CAD build for the part. Positions are in the model's coordinates, mm. Face numbers are marked on the shaded views. A direction names the side the tool comes from. Give positions to 0.01 mm unless a question says otherwise; leave off trailing zeros. Write each loop counter-clockwise with the first axis right and the second up, starting at its lowest first coordinate (ties: lowest second). Pieces come first, ordered by that corner, then holes. Notation, with made-up numbers: (8, 84) -> (43, 84) arc R23 cw to (43, 108) -> close; hole circle Ø11 at (-10.5, 48.5). An arc over 180 degrees is marked (long way). Answer as a JSON object with one key per item and string values.
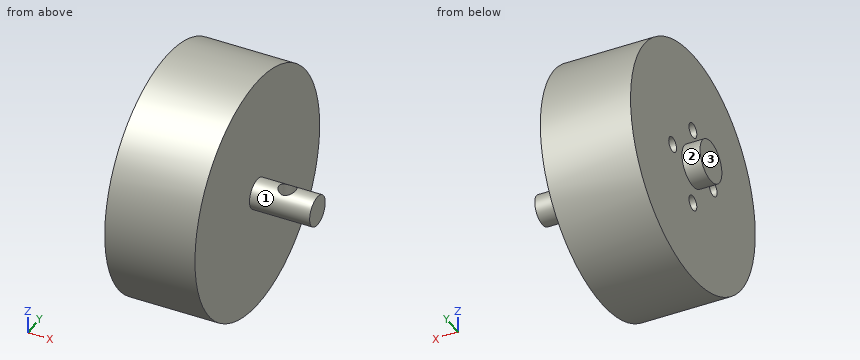
```python
from build123d import *

# Parameters (mm, degrees)
SKETCH_1_R               = 3.5
EXTRUDE_1_DEPTH          = 3
SKETCH_2_R               = 20
EXTRUDE_2_DEPTH          = 15
SKETCH_3_R               = 2.5
EXTRUDE_3_DEPTH          = 10
CUT_EXTRUDE_1_DEPTH      = 10
CUT_EXTRUDE_1_DEPTH_BACK = 10
SKETCH_4_R               = 1.4
HOLE_WIZARD_M3_1_D       = 2.5
HOLE_WIZARD_M3_1_DEPTH   = 6.748924226
HOLE_WIZARD_M3_1_TIP     = 0.751075774


with BuildPart() as part:
    # 草图1 → 凸台-拉伸1 (new body)
    with BuildSketch(Plane(origin=(0, 0, 0), x_dir=(0, 0, -1), z_dir=(1, 0, 0))):
        Circle(SKETCH_1_R)
    extrude(amount=EXTRUDE_1_DEPTH)

    # 草图2 → 凸台-拉伸2 (add)
    with BuildSketch(Plane(origin=(3, 0, 0), x_dir=(0, 0, -1), z_dir=(1, 0, 0))):
        Circle(SKETCH_2_R)
    extrude(amount=EXTRUDE_2_DEPTH)

    # 草图3 → 凸台-拉伸3 (add)
    with BuildSketch(Plane(origin=(18, 0, 0), x_dir=(0, 0, -1), z_dir=(1, 0, 0))):
        Circle(SKETCH_3_R)
    extrude(amount=EXTRUDE_3_DEPTH)

    # 草图4 → 切除-拉伸1 (cut, two sides: drawn at the far end of the back side and taken through both)
    with BuildSketch(Plane.XY.offset(-CUT_EXTRUDE_1_DEPTH_BACK)):
        with Locations((23, 0)):
            Circle(SKETCH_4_R)
    extrude(amount=CUT_EXTRUDE_1_DEPTH + CUT_EXTRUDE_1_DEPTH_BACK, mode=Mode.SUBTRACT)

    # M3 螺纹孔1
    with Locations(Plane(origin=(3, 0, 6.5), x_dir=(0, 0, -1), z_dir=(-1, 0, 0))):
        with Locations((0, 0), (6.5, 6.5), (13, 0), (6.5, -6.5)):
            Hole(HOLE_WIZARD_M3_1_D / 2, depth=HOLE_WIZARD_M3_1_DEPTH)
            with Locations((0, 0, -(HOLE_WIZARD_M3_1_DEPTH + HOLE_WIZARD_M3_1_TIP / 2))):  # 118° drill point
                Cone(0, HOLE_WIZARD_M3_1_D / 2, HOLE_WIZARD_M3_1_TIP, mode=Mode.SUBTRACT)


solid = part.part
```
1) Wall check: probe 1 along Y at (x, z) = (4.75, 0); probe 2 along Y at (x, z) = (8.75, 1); probe 3 along X at (y, z) = (6.5, 12.5). Give the ranges that are in metal, low to high.
Model answer:
{"probe 1": "y = -20 to -7.75, -5.25 to 5.25, 7.75 to 20", "probe 2": "y = -19.97 to -7.25, -5.75 to 5.75, 7.25 to 19.97", "probe 3": "x = 3 to 18"}
2) Slice it at B-B (y = 17.5). List the corners of the cut face in (x, z), then the cut area to 3 significant figures.
Model answer:
{"outline": "(3, -9.68) -> (18, -9.68) -> (18, 9.68) -> (3, 9.68) -> close", "area": "290 mm2"}
3) Pin check, flat tips, straight feed: pin 1 (4 mm diameter, centred on y = -6.5, z = 0, fed in from +X); pin 2 (4 mm diameter, centred on x = 15, z = 5, fed in from -Y); pin 3 (3 mm diameter, centred on y = 2, z = -9.5, fed in from -X). Stop position of each tip, or through.
Model answer:
{"pin 1": "stops at x = 18", "pin 2": "stops at y = -19.77", "pin 3": "stops at x = 3"}
4) 3-axis set-ups, long thin cutter, end or side, ignore diameter. For the marked faces 1, 2 and 3: which of +Z, -Z, +X, -X, +Y, -Y reach the whole face in a straight line?
Model answer:
{"face 1": "+X", "face 2": "-X", "face 3": "+Z, -Z, -X, +Y, -Y"}
5) Slice it at C-C (z = 8.5). List the corners of the cut face in (x, y), then the cut area to 3 significant figures.
Model answer:
{"outline": "(3, -18.1) -> (18, -18.1) -> (18, 18.1) -> (3, 18.1) -> close", "area": "543 mm2"}
6) Slice it at A-A (x = 22.5). List the corners of the cut face in (y, z), then the cut area to 3 significant figures.
Model answer:
{"outline": "(-1.31, -2.13) -> (-1.31, 2.13) arc R2.5 ccw to start; (1.31, -2.13) arc R2.5 ccw to (1.31, 2.13) -> close", "area": "7.18 mm2"}
